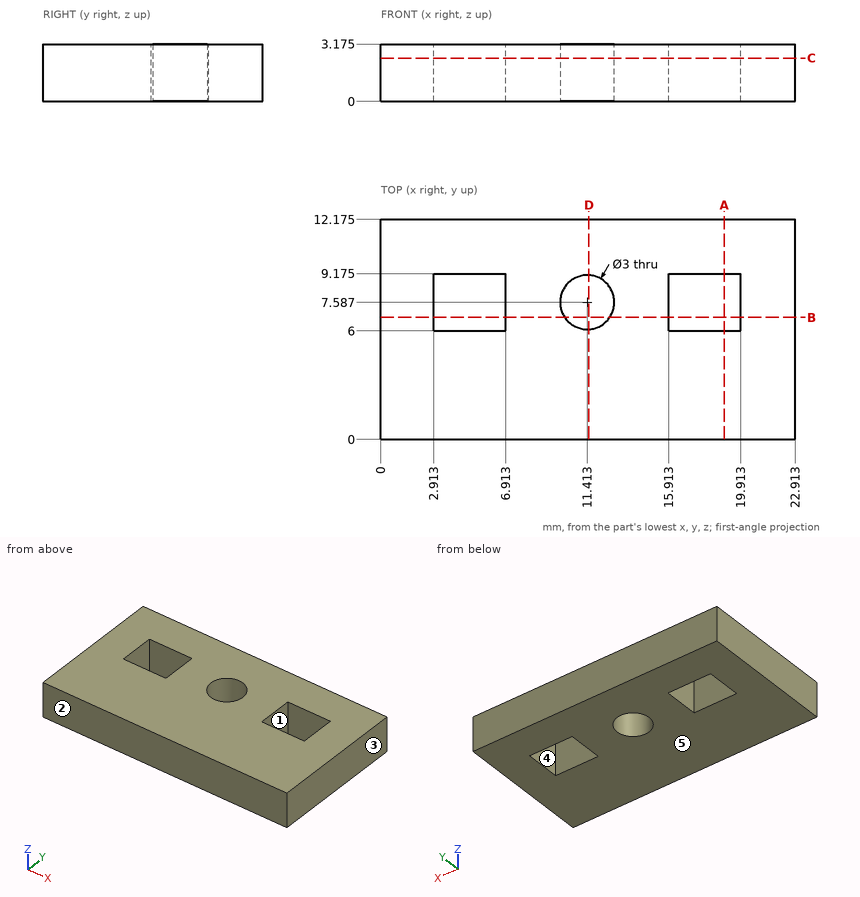
The drawing under review shows one solid part. Ordinate dimensions are in mm from its lowest x, y, z. A direction names the side the tool comes from. Give positions to 0.01 mm unless a question says otherwise; leave off trailing zeros. Order: outer loops, then holes, each group sorted by start corner. A loop starts at its lowest first (then second) coordinate and runs counter-clockwise, first axis right, second up. Notation, with made-up numbers: (-8, 56.5) - (40, 56.5) arc R16 ccw to (40, 86.5) - close; hole circle Ø6 at (39.25, 35). An arc over 180 degrees is marked (long way). Answer as a JSON object with one key per item and string values. Group by question number.
Item 1: Take a section at D-D on x = 11.5. Give the boundary of the cut face in (y, z) (1 decimal).
Item 2: Take a section at C-C on z = 2.4. Give the boundary of the cut face in (x, y) (1 decimal).
Item 3: Machinability: for the marked faces 4 and 5, which of the approach directions +Z, -Z, +X, -X, +Y, -Y give a long, thin tool a straight path to every point of the face, cutting with its end or side? Answer none if there is none.
Item 4: Take a section at A-A on x = 19. Give the boundary of the cut face in (y, z) (1 decimal).
Item 5: Draft analysis for pull direction X (two halves, no side actions). For the marked faces 1, 2 and 3, state which applies: pulls with the +X half, pulls with the -X half, needs draft (parallel to the pull), parting line crosses it, or undercut.
Item 6: Wall thickness on line 1 along X through (y, z) = (7.5, 0.75) (1 decimal); line 2 along Y through (x, z) = (6.5, 0.95) (1 decimal); line 3 along X through (y, z) = (7, 0.85): over which ranges is each line inside the solid? List them lowest first.
Item 7: Take a section at B-B on y = 6.75. Give the boundary of the cut face in (x, z) (1 decimal).
Reported:
{
 "1": {"outline": "(0, 0) - (6.1, 0) - (6.1, 3.2) - (0, 3.2) - close; (9.1, 0) - (12.2, 0) - (12.2, 3.2) - (9.1, 3.2) - close"},
 "2": {"outline": "(0, 0) - (22.9, 0) - (22.9, 12.2) - (0, 12.2) - close; hole (2.9, 6) - (6.9, 6) - (6.9, 9.2) - (2.9, 9.2) - close; hole circle Ø3 at (11.4, 7.6); hole (15.9, 6) - (19.9, 6) - (19.9, 9.2) - (15.9, 9.2) - close"},
 "3": {"face 4": "+Z, -Z", "face 5": "-Z, +X, -X, +Y, -Y"},
 "4": {"outline": "(0, 0) - (6, 0) - (6, 3.2) - (0, 3.2) - close; (9.2, 0) - (12.2, 0) - (12.2, 3.2) - (9.2, 3.2) - close"},
 "5": {"face 1": "undercut", "face 2": "needs draft", "face 3": "pulls with the +X half"},
 "6": {"line 1": "0 to 2.9, 6.9 to 9.9, 12.9 to 15.9, 19.9 to 22.9", "line 2": "0 to 6, 9.2 to 12.2", "line 3": "0 to 2.91, 6.91 to 10.03, 12.79 to 15.91, 19.91 to 22.91"},
 "7": {"outline": "(0, 0) - (2.9, 0) - (2.9, 3.2) - (0, 3.2) - close; (6.9, 0) - (10.2, 0) - (10.2, 3.2) - (6.9, 3.2) - close; (12.7, 0) - (15.9, 0) - (15.9, 3.2) - (12.7, 3.2) - close; (19.9, 0) - (22.9, 0) - (22.9, 3.2) - (19.9, 3.2) - close"}
}
